```python
from build123d import *

# Parameters (mm, degrees)
SALIENTE_EXTRUIR1_DEPTH = 7
CROQUIS2_R              = 1.125
CORTAR_EXTRUIR1_DEPTH   = 10
CROQUIS4_R              = 1.125
CORTAR_EXTRUIR2_DEPTH   = 10
CROQUIS5_R              = 1.125
CORTAR_EXTRUIR3_DEPTH   = 10
REDONDEO1_R             = 10
REDONDEO2_R             = 0.5
REDONDEO3_R             = 1
CORTAR_EXTRUIR4_DEPTH   = 10
REDONDEO4_R             = 3
REDONDEO5_R             = 1
CHAFL_N1_SIZE           = 2


with BuildPart() as part:
    # Croquis1 → Saliente-Extruir1 (new body)
    with BuildSketch(Plane(origin=(0, 0, 0), x_dir=(1, 0, 0), z_dir=(0, 1, 0))):
        Polygon((34.641016151, 0), (17.320508076, 30), (-17.320508076, 30), (-34.641016151, 0), (-17.320508076, -30), (17.320508076, -30), align=None)
    extrude(amount=SALIENTE_EXTRUIR1_DEPTH)

    # Croquis2 → Cortar-Extruir1 (cut)
    with BuildSketch(Plane(origin=(25.980762114, 0, 15), x_dir=(0.5, 0, -0.866025404), z_dir=(0.866025404, 0, 0.5))):
        with Locations((0, 3.5)):
            Circle(CROQUIS2_R)
    extrude(amount=-CORTAR_EXTRUIR1_DEPTH, mode=Mode.SUBTRACT)

    # Croquis4 → Cortar-Extruir2 (cut)
    with BuildSketch(Plane(origin=(-25.980762114, 0, 15), x_dir=(0.5, 0, 0.866025404), z_dir=(-0.866025404, 0, 0.5))):
        with Locations((0, 3.5)):
            Circle(CROQUIS4_R)
    extrude(amount=-CORTAR_EXTRUIR2_DEPTH, mode=Mode.SUBTRACT)

    # Croquis5 → Cortar-Extruir3 (cut)
    with BuildSketch(Plane(origin=(0, 0, -30), x_dir=(-1, 0, 0), z_dir=(0, 0, -1))):
        with Locations((0, 3.5)):
            Circle(CROQUIS5_R)
    extrude(amount=-CORTAR_EXTRUIR3_DEPTH, mode=Mode.SUBTRACT)

    # Redondeo1
    redondeo1_edges = [part.edges().sort_by_distance(p)[0] for p in [
        (17.320508076, 3.5, 30),
        (-17.320508076, 3.5, 30),
        (-34.641016151, 3.5, 0),
        (-17.320508076, 3.5, -30),
        (17.320508076, 3.5, -30),
        (34.641016151, 3.5, 0),
    ]]
    fillet(redondeo1_edges, radius=REDONDEO1_R)

    # Redondeo2
    redondeo2_edges = [part.edges().sort_by_distance(p)[0] for p in [
        (25.418262114, 3.5, 15.974278579),
        (-26.543262114, 3.5, 14.025721421),
        (1.125, 3.5, -30),
    ]]
    fillet(redondeo2_edges, radius=REDONDEO2_R)

    # Redondeo3
    redondeo3_edges = [part.edges().sort_by_distance(p)[0] for p in [
        (25.980762114, 7, 15),
        (0, 7, 30),
        (25.980762114, 7, -15),
        (0, 7, -30),
        (-25.980762114, 7, -15),
        (-25.980762114, 7, 15),
        (-16.547005384, 7, -28.660254038),
        (-33.094010768, 7, 0),
        (-16.547005384, 7, 28.660254038),
        (16.547005384, 7, -28.660254038),
        (33.094010768, 7, 0),
        (16.547005384, 7, 28.660254038),
    ]]
    fillet(redondeo3_edges, radius=REDONDEO3_R)

    # Croquis6 → Cortar-Extruir4 (cut)
    with BuildSketch(Plane(origin=(0, 7, 0), x_dir=(1, 0, 0), z_dir=(0, 1, 0))):
        Polygon((-15.529142706, 0), (-13.448632083, -7.764571353), (-7.764571353, -13.448632083), (0, -15.529142706), (7.764571353, -13.448632083), (13.448632083, -7.764571353), (15.529142706, 0), (13.448632083, 7.764571353), (7.764571353, 13.448632083), (0, 15.529142706), (-7.764571353, 13.448632083), (-13.448632083, 7.764571353), align=None)
    extrude(amount=-CORTAR_EXTRUIR4_DEPTH, mode=Mode.SUBTRACT)

    # Redondeo4
    redondeo4_edges = [part.edges().sort_by_distance(p)[0] for p in [
        (-14.488887394, 7, -3.882285677),
        (-14.488887394, 7, 3.882285677),
        (-10.606601718, 7, 10.606601718),
        (-3.882285677, 7, 14.488887394),
        (3.882285677, 7, 14.488887394),
        (10.606601718, 7, 10.606601718),
        (14.488887394, 7, 3.882285677),
        (14.488887394, 7, -3.882285677),
        (10.606601718, 7, -10.606601718),
        (3.882285677, 7, -14.488887394),
        (-3.882285677, 7, -14.488887394),
        (-10.606601718, 7, -10.606601718),
    ]]
    fillet(redondeo4_edges, radius=REDONDEO4_R)

    # Redondeo5
    redondeo5_edges = [part.edges().sort_by_distance(p)[0] for p in [
        (25.980762114, 0, 15),
        (0, 0, 30),
        (-25.980762114, 0, 15),
        (-25.980762114, 0, -15),
        (0, 0, -30),
        (25.980762114, 0, -15),
        (-16.547005384, 0, -28.660254038),
        (-33.094010768, 0, 0),
        (-16.547005384, 0, 28.660254038),
        (16.547005384, 0, -28.660254038),
        (33.094010768, 0, 0),
        (16.547005384, 0, 28.660254038),
    ]]
    fillet(redondeo5_edges, radius=REDONDEO5_R)

    # Chaflán1
    chafl_n1_edges = [part.edges().sort_by_distance(p)[0] for p in [
        (-14.488887394, 0, 3.882285677),
        (-10.606601718, 0, 10.606601718),
        (-3.882285677, 0, 14.488887394),
        (3.882285677, 0, 14.488887394),
        (10.606601718, 0, 10.606601718),
        (14.488887394, 0, 3.882285677),
        (14.488887394, 0, -3.882285677),
        (10.606601718, 0, -10.606601718),
        (3.882285677, 0, -14.488887394),
        (-3.882285677, 0, -14.488887394),
        (-10.606601718, 0, -10.606601718),
        (-14.488887394, 0, -3.882285677),
    ]]
    chamfer(chafl_n1_edges, length=CHAFL_N1_SIZE)


solid = part.part
```
The listing builds one solid part. Answer for the finished solid, in the listing's coordinates (mm). A direction names the side the tool comes from. Coordinates: 2 decimals unless noted, no trailing zeros. Answer as a JSON object with one key per item and string values. Group by question number.
Item 1: Consider L1, parallel to Y at x = 0, z = -22.25 (3 decimals); L2, parallel to Z at x = -13, y = 2.25; L3, parallel to Z at x = -10.5, y = 1.25. Determine where each line is inside the solid, lowest interval first.
Item 2: Which of the six approach directions +Z, -Z, +X, -X, +Y, -Y give full straight-line access (tool end or side, diameter ignored) to faces 5 (the face through (10.646, 3.014, -10.567)), 6 (the face through (-21.19, 4.45, 12.93)), 7 (the face through (4.08, 1.01, 15.46)), 8 (the face through (4.18, 6.14, 15.34))?
Item 3: Each of these flat-tipped pins is pushed along its axis until it touches: P1, Ø3, axis at y = 5, z = 6.5, coming from the +X side; P2, Ø1.8, axis at x = 0, y = 3.5, coming from the -Z side; P3, Ø2, axis at y = 3, z = 2, coming from the +X side. Where does it stop, or does it pass through?
Item 4: Determine the mould class of faces 1 (the face through (-15.46, 1.01, 4.08)), 2 (the face through (33.094, 3.535, -0.073)), 3 (the face through (-10.646, 3.014, 10.567)), 4 (the face through (0, 3, 30)) for opening direction X: +X half, -X half, draft (parallel to the pull), parting line (faces both ways), or undercut.
Solved:
{
 "1": {"L1": "y = 0 to 2.375, 4.625 to 7", "L2": "z = -29.89 to -8.21, 8.21 to 29.89", "L3": "z = -30 to -11.77, 11.77 to 30"},
 "2": {"face 5": "+Y, -Y", "face 6": "none", "face 7": "-Y", "face 8": "+Y"},
 "3": {"P1": "stops at x = 31.75", "P2": "stops at z = -20", "P3": "stops at x = 33.04"},
 "4": {"face 1": "undercut", "face 2": "+X half", "face 3": "undercut", "face 4": "draft"}
}
